Geometry check sheet. Reference: the model listing, model coordinates, mm. Face numbers are marked on the shaded views. A direction names the side the tool comes from. Give positions to 0.01 mm unless a question says otherwise; leave off trailing zeros. Loops run counter-clockwise (first coordinate to the right, second up) from the corner with the lowest first, then second, coordinate; pieces in that order, holes last.
1. Cross-section at C-C, the plane z = 5.5. Record the cut outline in (x, y), plus the area to 3 significant figures.
2. Tool access check on the marked faces 1, 2, 3 and 4. Record the directions out of +Z, -Z, +X, -X, +Y, -Y that give a thin tool (end or side, any length) a straight path to the whole face; none if there is none.
3. Cross-section at D-D, the plane x = 6. Record the cut outline in (y, z).
4. Cross-section at B-B, the plane x = 15.7. Record the cut outline in (y, z), plus the area to 3 significant figures.
5. Cross-section at A-A, the plane z = 22.5. Record the cut outline in (x, y).
6. Release check for a two-part mould opening along Y. For the marked faces 5, 6 and 7 record: +Y half, -Y half, draft (parallel to the pull), parting line (faces both ways), or undercut.
7. Go/stop test with flat-tipped pins: pin 1 Ø1.9 at (y, z) = (1, 14.5) entering from +X; pin 2 Ø3 at (x, z) = (-15.7, 6) entering from +Y; pin 3 Ø12 at (y, z) = (9.5, 15.5) entering from -X; pin 4 Ø1 at (x, y) = (0.5, -3.5) entering from +Z. Record where each tip stops, or that it passes through.
8. Material ranges on L1, parallel to X at y = -1.25, z = 6; L2, parallel to Y at x = -6, z = 19; L3, parallel to Y at x = 5.5, z = 24, recorded low to high.
from build123d import *

# Parameters (mm, degrees)
F1_DEPTH = 7.25
F0_W     = 24
F0_H     = 8
F2_DEPTH = 1.7
F4_DEPTH = 10
F6_DEPTH = 3.5
F7_R     = 5
F9_D     = 3.6


with BuildPart() as f1:
    # F0 (on Front) → F1 (new body)
    with BuildSketch(Plane.XZ):
        with BuildLine():
            Line((20, 12), (12, 12))
            ThreePointArc((12, 12), (8.4852813844, 3.5147186359), (2.86e-08, 0))
            Line((2.86e-08, 0), (20, 0))
            Line((20, 0), (20, 12))
        make_face()
        with BuildLine():
            Line((12, 12), (-12, 12))
            ThreePointArc((-12, 12), (-8.4852813641, 3.5147186156), (2.86e-08, 0))
            ThreePointArc((2.86e-08, 0), (8.4852813844, 3.5147186359), (12, 12))
        make_face()
        with BuildLine():
            Line((-12, 12), (-20, 12))
            Line((-20, 12), (-20, 0))
            Line((-20, 0), (2.86e-08, 0))
            ThreePointArc((2.86e-08, 0), (-8.4852813641, 3.5147186156), (-12, 12))
        make_face()
    extrude(amount=F1_DEPTH)



with BuildPart() as f1b:
    # F0 (on Front) → F1, piece 2 (new body)
    with BuildSketch(Plane.XZ):
        with BuildLine():
            ThreePointArc((12, 20), (0, 32), (-12, 20))
            Line((-12, 20), (12, 20))
        make_face()
    extrude(amount=F1_DEPTH)


with BuildPart() as f1_1:
    add(f1.part)

    add(f1b.part)  # F2 merges F1b
    # F0 (on Front) → F2 (join)
    with BuildSketch(Plane.XZ):
        with BuildLine():
            ThreePointArc((12, 20), (0, 32), (-12, 20))
            Line((-12, 20), (12, 20))
        make_face()
        with Locations((0, 16)):
            Rectangle(F0_W, F0_H)
        with BuildLine():
            Line((12, 12), (-12, 12))
            ThreePointArc((-12, 12), (-8.4852813641, 3.5147186156), (2.86e-08, 0))
            ThreePointArc((2.86e-08, 0), (8.4852813844, 3.5147186359), (12, 12))
        make_face()
    extrude(amount=-F2_DEPTH)

    # F3 (on face) → F4 (join)
    with BuildSketch(Plane(origin=(0, 1.7, 0), x_dir=(-1, 0, 0), z_dir=(0, 1, 0))):
        with BuildLine():
            ThreePointArc((-12, 12), (0, 0), (12, 12))
            Line((12, 12), (-12, 12))
        make_face()
    extrude(amount=F4_DEPTH)

    # F5 (on face) → F6 (join)
    with BuildSketch(Plane(origin=(0, 11.7, 0), x_dir=(-1, 0, 0), z_dir=(0, 1, 0))):
        with BuildLine():
            ThreePointArc((12, 20), (0, 32), (-12, 20))
            Line((-12, 20), (-12, 12))
            ThreePointArc((-12, 12), (0, 0), (12, 12))
            Line((12, 12), (12, 20))
        make_face()
    extrude(amount=F6_DEPTH)

    # F7
    f7_edges = [f1_1.edges().sort_by_distance(p)[0] for p in [
        (-20, -3.625, 12),
        (-20, -3.625, 0),
        (20, -3.625, 12),
        (20, -3.625, 0),
    ]]
    fillet(f7_edges, radius=F7_R)

    # F9 (through all)
    with Locations(Plane(origin=(0, 0, 0), x_dir=(1, 0, 0), z_dir=(0, 1, 0))):
        with Locations((15.7, -6), (-15.7, -6)):
            Hole(F9_D / 2)


solid = f1_1.part
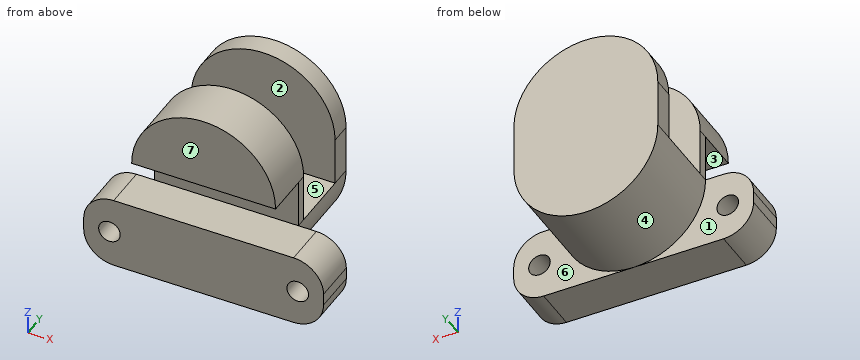
Result:
1. outline: (-20, -7.25) - (-17.43, -7.25) - (-17.43, 0) - (-20, 0) - close; (-13.97, -7.25) - (13.97, -7.25) - (13.97, 0) - (10.09, 0) - (10.09, 15.2) - (-10.09, 15.2) - (-10.09, 0) - (-13.97, 0) - close; (17.43, -7.25) - (20, -7.25) - (20, 0) - (17.43, 0) - close
1. area: 547 mm2
2. face 1: -Z, -X, +Y
2. face 2: +Z, +X, -X
2. face 3: +X, -X, -Y
2. face 4: -Z, +Y
3. outline: (-7.25, 0) - (0, 0) - (0, 1.61) - (15.2, 1.61) - (15.2, 30.39) - (11.7, 30.39) - (11.7, 12) - (1.7, 12) - (1.7, 30.39) - (-7.25, 30.39) - (-7.25, 20) - (0, 20) - (0, 12) - (-7.25, 12) - close
4. outline: (-7.25, 0.05) - (0, 0.05) - (0, 4.2) - (-7.25, 4.2) - close; (-7.25, 7.8) - (0, 7.8) - (0, 11.95) - (-7.25, 11.95) - close
4. area: 60.2 mm2
5. outline: (-11.74, -7.25) - (11.74, -7.25) - (11.74, 1.7) - (-11.74, 1.7) - close; (-11.74, 11.7) - (11.74, 11.7) - (11.74, 15.2) - (-11.74, 15.2) - close
6. face 5: undercut
6. face 6: +Y half
6. face 7: -Y half
7. pin 1: stops at x = 12
7. pin 2: passes through
7. pin 3: stops at x = -12
7. pin 4: stops at z = 32
8. L1: x = -20 to -17.5, -13.9 to 13.9, 17.5 to 20
8. L2: y = 0 to 1.7, 11.7 to 15.2
8. L3: y = -7.25 to 1.7, 11.7 to 15.2
